```python
from build123d import *

# Parameters (mm, degrees)
F2_R = 0.254
F3_R = 0.254


with BuildPart() as f1:
    # F0 (on Front) → F1 (revolve)
    with BuildSketch(Plane.XZ):
        Polygon((6.3627, 0), (0, 0), (0, -3.175), (69.85, -3.175), (69.85, 1.5875), (63.5, 1.5875), (63.5, 0), (7.9375, 0), (7.9375, -0.508), (6.3627, -0.508), align=None)
    revolve(axis=Axis((34.925, 0, -3.175), (-1, 0, 0)))

    # F2
    f2_edges = [f1.edges().sort_by_distance(p)[0] for p in [
        (0, 0, -6.35),
        (63.5, 0, -7.9375),
        (69.85, 0, -7.9375),
    ]]
    fillet(f2_edges, radius=F2_R)

    # F3
    f3_edges = [f1.edges().sort_by_distance(p)[0] for p in [
        (7.9375, 0, -6.35),
        (6.3627, 0, -6.35),
    ]]
    fillet(f3_edges, radius=F3_R)


solid = f1.part
```
CAD build for the part. Positions are in the model's coordinates, mm. A direction names the side the tool comes from. Coordinates: 2 decimals unless noted, no trailing zeros. Loops run counter-clockwise (first coordinate to the right, second up) from the corner with the lowest first, then second, coordinate; pieces in that order, holes last. Notation, with made-up numbers: (-4, 76) - (5, 76) arc R9 cw to (5, 87) - close; hole circle Ø8 at (-28.5, 66). An arc over 180 degrees is marked (long way). Return JSON: item names as keys, results as strings.
1. 3-axis set-ups, long thin cutter, end or side, ignore diameter. For faces 1 (the cylindrical face through (35.459, 0.954, -0.147)), 2 (the flat face through (0, 0, -3)): which of +Z, -Z, +X, -X, +Y, -Y reach the whole face in a straight line?
Result:
{"face 1": "-X", "face 2": "+Z, -Z, -X, +Y, -Y"}
2. Probe L1, parallel to X at y = 0.5, z = -0.5; L2, parallel to Y at x = 20.5, z = -3.25; L3, parallel to X at y = 3.25, z = -3.5. List the from-to ranges inside material, lowest first. Write a range as from..to.
Result:
{"L1": "x = 0..6.36, 7.94..69.85", "L2": "y = -3.17..3.17", "L3": "x = 63.5..69.85"}
3. Band-saw the part on B-B (x = 42). Give the cut face in (y, z) (3 decimals).
Result:
{"outline": "circle Ø6.35 at (0, -3.175)"}
4. Mould opens along X. For faces 3 (the cylindrical face through (66.634, 0.209, -7.933)), 4 (the flat face through (63.5, -3, -1)), 5 (the flat face through (69.85, 0, -3)), 6 (the cylindrical face through (7.14, 0.8, -0.63)) say: released by +X, released by -X, zero draft, split by the parting line, or undercut.
Result:
{"face 3": "zero draft", "face 4": "released by -X", "face 5": "released by +X", "face 6": "undercut"}
5. Drop flat-ended pins along their axis: pin 1 (4 mm diameter, centred on x = 27.5, z = -5.5, fed in from -Y); pin 2 (3 mm diameter, centred on y = 0.5, z = -3, fed in from -X); pin 3 (1.5 mm diameter, centred on x = 54, y = 3, fed in from -Z); pin 4 (2 mm diameter, centred on x = 52.5, y = 3, fed in from -Z). Give the stop position or say it passes through.
Result:
{"pin 1": "stops at y = -3.16", "pin 2": "stops at x = 0", "pin 3": "stops at z = -5.42", "pin 4": "stops at z = -5.64"}
6. Band-saw the part on A-A (y = 0). Give the cut face in (x, z), and give its area (3 significant figures).
Result:
{"outline": "(0, -6.1) arc R0.25 ccw to (0.25, -6.35) - (6.11, -6.35) arc R0.25 ccw to (6.36, -6.1) - (6.36, -5.84) - (7.94, -5.84) - (7.94, -6.1) arc R0.25 ccw to (8.19, -6.35) - (63.5, -6.35) - (63.5, -7.68) arc R0.25 ccw to (63.75, -7.94) - (69.6, -7.94) arc R0.25 ccw to (69.85, -7.68) - (69.85, 1.33) arc R0.25 ccw to (69.6, 1.59) - (63.75, 1.59) arc R0.25 ccw to (63.5, 1.33) - (63.5, 0) - (8.19, 0) arc R0.25 ccw to (7.94, -0.25) - (7.94, -0.51) - (6.36, -0.51) - (6.36, -0.25) arc R0.25 ccw to (6.11, 0) - (0.25, 0) arc R0.25 ccw to (0, -0.25) - close", "area": "462 mm2"}
